Design review of the part built by this model. Coordinates are the model's own, in mm. A direction names the side the tool comes from. Give positions to 0.01 mm unless a question says otherwise; leave off trailing zeros. Write each loop counter-clockwise with the first axis right and the second up, starting at its lowest first coordinate (ties: lowest second). Pieces come first, ordered by that corner, then holes.
```python
from build123d import *

# Parameters (mm, degrees)
F0_R     = 25.4
F2_DEPTH = 38.1
F0_W     = 38.354
F0_H     = 38.1
F3_DEPTH = 25.4


# Not quite as in the source:
# - a variable given as a bare number and used for a length is read in inches; the dataset says mm whatever the document's units were


with BuildPart() as f2:
    # F0 (on Top) → F2 (new body)
    with BuildSketch(Plane.XY):
        with BuildLine():
            ThreePointArc((-76.2, 571.9231766592), (-355.0918394716, 205.012369106), (-533.4, -219.9704525612))
            Line((-533.4, -219.9704525612), (-504.8885, -269.3538191612))
            Line((-504.8885, -269.3538191612), (-471.8929321158, -250.3038191612))
            Line((-471.8929321158, -250.3038191612), (-452.7159321158, -283.519357498))
            Line((-452.7159321158, -283.519357498), (-485.7115, -302.569357498))
            Line((-485.7115, -302.569357498), (-457.2, -351.952724098))
            ThreePointArc((-457.2, -351.952724098), (0, -401.5140680266), (457.2, -351.952724098))
            Line((457.2, -351.952724098), (485.7115, -302.569357498))
            Line((485.7115, -302.569357498), (452.7159321158, -283.519357498))
            Line((452.7159321158, -283.519357498), (471.8929321158, -250.3038191612))
            Line((471.8929321158, -250.3038191612), (504.8885, -269.3538191612))
            Line((504.8885, -269.3538191612), (533.4, -219.9704525612))
            ThreePointArc((533.4, -219.9704525612), (347.7213828878, 200.7570340133), (76.2, 571.9231766592))
            Line((76.2, 571.9231766592), (19.177, 571.9231766592))
            Line((19.177, 571.9231766592), (19.177, 533.8231766592))
            Line((19.177, 533.8231766592), (-19.177, 533.8231766592))
            Line((-19.177, 533.8231766592), (-19.177, 571.9231766592))
            Line((-19.177, 571.9231766592), (-76.2, 571.9231766592))
        make_face()
        with Locations((-407.3118189755, -235.1615883296)):
            Circle(F0_R, mode=Mode.SUBTRACT)
        Polygon((-21.9970452561, 38.1), (21.9970452561, 38.1), (43.9940905122, 0), (21.9970452561, -38.1), (-21.9970452561, -38.1), (-43.9940905122, 0), align=None, mode=Mode.SUBTRACT)
        with Locations((407.3118189755, -235.1615883296)):
            Circle(F0_R, mode=Mode.SUBTRACT)
        with Locations((0, 470.3231766592)):
            Circle(F0_R, mode=Mode.SUBTRACT)
    extrude(amount=F2_DEPTH)

    # F0 (on Top) → F3 (join)
    with BuildSketch(Plane.XY):
        Polygon((-471.8929321158, -250.3038191612), (-504.8885, -269.3538191612), (-485.7115, -302.569357498), (-452.7159321158, -283.519357498), align=None)
        Polygon((452.7159321158, -283.519357498), (485.7115, -302.569357498), (504.8885, -269.3538191612), (471.8929321158, -250.3038191612), align=None)
        with Locations((0, 552.8731766592)):
            Rectangle(F0_W, F0_H)
    extrude(amount=F3_DEPTH)


solid = f2.part
```
(1) To check wall thickness, follow L1, parallel to X at y = -218, z = 11; L2, parallel to X at y = -256.5, z = 15.5; L3, parallel to X at y = 492, z = 24. State the ranges of each line that lie inside material, in increasing order.
Resolved:
L1: x = -532.85 to -426.04, -388.59 to 388.59, 426.04 to 532.77
L2: x = -512.31 to -421.09, -393.53 to 393.53, 421.09 to 512.31
L3: x = -150.14 to -13.24, 13.24 to 145.56
(2) Consider section B-B, the plane z = 16. Give the boundary of the cut face in (x, y).
Resolved:
outline: (-533.4, -219.97) - (-457.2, -351.95) arc R2133.6 ccw to (457.2, -351.95) - (533.4, -219.97) arc R2133.6 ccw to (76.2, 571.92) - (-76.2, 571.92) arc R1828.8 ccw to start; hole circle Ø50.8 at (-407.31, -235.16); hole (-43.99, 0) - (-22, -38.1) - (22, -38.1) - (43.99, 0) - (22, 38.1) - (-22, 38.1) - close; hole circle Ø50.8 at (0, 470.32); hole circle Ø50.8 at (407.31, -235.16)
(3) Tool access review of faces 4 (the face through (-479, -276, 25.4)), 5 (the face through (0, 553, 25.4)), 6 (the face through (-32.84, -19.32, 18.78)): name each direction out of +Z, -Z, +X, -X, +Y, -Y from which nothing blocks a thin tool from reaching the whole face with its end or side.
Resolved:
face 4: +Z
face 5: +Z, +Y
face 6: +Z, -Z
(4) Clearance check with flat-ended pins moving along their axes: P1, Ø10, axis at y = 559, z = 33, coming from the -X side; P2, Ø4, axis at y = -152.5, z = 11, coming from the -X side; P3, Ø6, axis at y = 405.5, z = 31, coming from the +X side. State where each tip first meets the part, or that it passes through.
Resolved:
P1: stops at x = -93.56
P2: stops at x = -513.89
P3: stops at x = 215.5
(5) Consider section A-A, the plane x = 0. Give the boundary of the cut face in (y, z), then the cut area to 3 significant figures.
Resolved:
outline: (-401.51, 0) - (-38.1, 0) - (-38.1, 38.1) - (-401.51, 38.1) - close; (38.1, 0) - (444.92, 0) - (444.92, 38.1) - (38.1, 38.1) - close; (495.72, 0) - (571.92, 0) - (571.92, 25.4) - (533.82, 25.4) - (533.82, 38.1) - (495.72, 38.1) - close
area: 31,800 mm2
(6) Consider section D-D, the plane x = 286. Give the boundary of the cut face in (y, z), then the cut area to 3 significant figures.
Resolved:
outline: (-382.26, 0) - (301.15, 0) - (301.15, 38.1) - (-382.26, 38.1) - close
area: 26,000 mm2
(7) Mouldability with a two-part tool opening along X and no side actions: class faces 1 (the face through (-7, 92, 38.1)), 2 (the face through (-351.847, 210.609, 18.783)), 3 (the face through (0, 38.1, 19)) as pulls with the +X half, pulls with the -X half, needs draft (parallel to the pull), parting line crosses it, or undercut.
Resolved:
face 1: needs draft
face 2: pulls with the -X half
face 3: undercut
(8) Consider section C-C, the plane y = 248. Give the boundary of the cut face in (x, z).
Resolved:
outline: (-329.48, 0) - (319.63, 0) - (319.63, 38.1) - (-329.48, 38.1) - close
